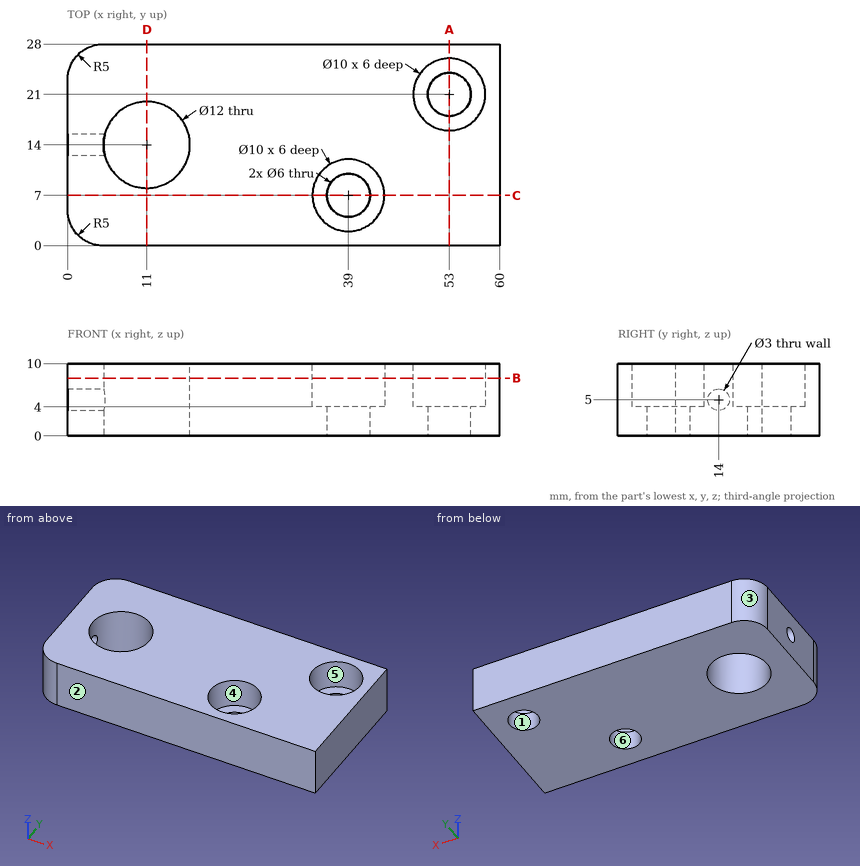
Design review of the part shown in the three views and the two pictorial views. Dimensions are in mm from the part's minimum x, y and z. A direction names the side the tool comes from. Round coordinates to 2 decimals unless told otherwise and drop trailing zeros. Loops run counter-clockwise (first coordinate to the right, second up) from the corner with the lowest first, then second, coordinate; pieces in that order, holes last.
1) Consider section B-B on z = 8. State the section outline as (x, y) points.
Values follow:
outline: (0, 5) arc R5 ccw to (5, 0) - (60, 0) - (60, 28) - (5, 28) arc R5 ccw to (0, 23) - close; hole circle Ø12 at (11, 14); hole circle Ø10 at (39, 7); hole circle Ø10 at (53, 21)
2) Clearance check with flat-ended pins moving along their axes: P1, Ø7, axis at x = 39, y = 7, coming from the +Z side; P2, Ø5, axis at x = 53, y = 21, coming from the -Z side. State where each tip first meets the part, or that it passes through.
Values follow:
P1: stops at z = 4
P2: passes through
3) Consider section A-A on x = 53. State the section outline as (y, z) points, then the cut area to 3 significant figures.
Values follow:
outline: (0, 0) - (18, 0) - (18, 4) - (16, 4) - (16, 10) - (0, 10) - close; (24, 0) - (28, 0) - (28, 10) - (26, 10) - (26, 4) - (24, 4) - close
area: 196 mm2
4) Tool access review of the marked faces 5 and 6: name each direction out of +Z, -Z, +X, -X, +Y, -Y from which nothing blocks a thin tool from reaching the whole face with its end or side.
Values follow:
face 5: +Z
face 6: +Z, -Z
5) Consider section D-D on x = 11. State the section outline as (y, z) points, then the cut area to 3 significant figures.
Values follow:
outline: (0, 0) - (8, 0) - (8, 10) - (0, 10) - close; (20, 0) - (28, 0) - (28, 10) - (20, 10) - close
area: 160 mm2
6) Wall thickness on line 1 along Z through (x, y) = (3.9, 14); line 2 along Y through (x, z) = (39, 2.4); line 3 along X through (y, z) = (18.75, 7.5): over which ranges is each line inside the solid? List them lowest first.
Values follow:
line 1: z = 0 to 3.5, 6.5 to 10
line 2: y = 0 to 4, 10 to 28
line 3: x = 0 to 7.33, 14.67 to 48.53, 57.47 to 60
7) The part is to be moulded in two halves that separate along X. For the marked faces 1, 2, 3 and 4, say which applies: pulls with the +X half, pulls with the -X half, needs draft (parallel to the pull), parting line crosses it, or undercut.
Values follow:
face 1: undercut
face 2: needs draft
face 3: pulls with the -X half
face 4: undercut
8) Consider section C-C on y = 7. State the section outline as (x, z) points, then the cut area to 3 significant figures.
Values follow:
outline: (0, 0) - (36, 0) - (36, 4) - (34, 4) - (34, 10) - (0, 10) - close; (42, 0) - (60, 0) - (60, 10) - (44, 10) - (44, 4) - (42, 4) - close
area: 516 mm2
